Input: part model. Units: mm. Frame: model coordinates. Face numbers are marked on the shaded views. A direction names the side the tool comes from. Round coordinates to 2 decimals unless told otherwise and drop trailing zeros. Write each loop counter-clockwise with the first axis right and the second up, starting at its lowest first coordinate (ties: lowest second). Pieces come first, ordered by that corner, then holes. Notation, with made-up numbers: (57.5, 28) -> (77.5, 28) arc R24 ccw to (77.5, 59) -> close; hole circle Ø4 at (-30.5, -4.75). An arc over 180 degrees is marked (long way). Use CSV: the item, a comma, the result in double quotes.
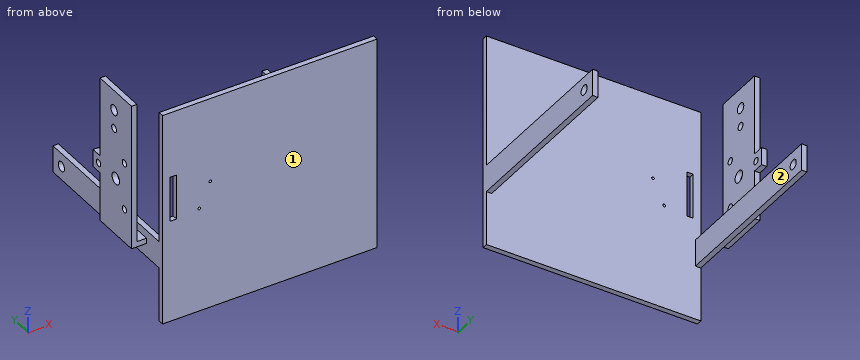
```python
from build123d import *

# Parameters (mm, degrees)
SKETCH1_W                 = 199
SKETCH1_H                 = 199
BOSS_EXTRUDE1_DEPTH       = 5
SKETCH2_W                 = 5
SKETCH2_H                 = 25
BOSS_EXTRUDE2_DEPTH       = 18.8
SKETCH3_W                 = 5
SKETCH3_H                 = 25
BOSS_EXTRUDE3_DEPTH       = 46.4
SKETCH4_W                 = 5
SKETCH4_H                 = 25
BOSS_EXTRUDE4_DEPTH       = 91.8
SKETCH5_W                 = 5
SKETCH5_H                 = 25
BOSS_EXTRUDE5_DEPTH       = 157
SKETCH6_R                 = 4.5
CUT_EXTRUDE1_DEPTH        = 325.724498614
SKETCH8_W                 = 5
SKETCH8_H                 = 46.4
BOSS_EXTRUDE6_DEPTH       = 13.9
SKETCH9_W                 = 5
SKETCH9_H                 = 46.4
BOSS_EXTRUDE7_DEPTH       = 131
SKETCH11_W                = 16.3
SKETCH11_H                = 10.35
BOSS_EXTRUDE8_DEPTH       = 5
SKETCH10_R                = 5.5
SKETCH10_R_2              = 3.15
CUT_EXTRUDE2_DEPTH        = 5
SKETCH12_W                = 6
SKETCH12_H                = 42
CUT_EXTRUDE3_DEPTH        = 5
SKETCH17_R                = 3.5
CUT_EXTRUDE7_DEPTH        = 9
M3X0_5_TAPPED_HOLE1_D     = 2.5
M3X0_5_TAPPED_HOLE1_DEPTH = 7.5
M3X0_5_TAPPED_HOLE1_TIP   = 0.751075774
SKETCH20_R                = 4.7625
CUT_EXTRUDE8_DEPTH        = 10


with BuildPart() as part:
    # Sketch1 → Boss-Extrude1 (new body)
    with BuildSketch(Plane(origin=(0, 0, 0), x_dir=(1, 0, 0), z_dir=(0, 1, 0))):
        with Locations((99.5, -99.5)):
            Rectangle(SKETCH1_W, SKETCH1_H)
    extrude(amount=BOSS_EXTRUDE1_DEPTH)

    # Sketch2 → Boss-Extrude2 (add)
    with BuildSketch(Plane(origin=(0, 5, 0), x_dir=(1, 0, 0), z_dir=(0, 1, 0))):
        with Locations((2.5, -63)):
            Rectangle(SKETCH2_W, SKETCH2_H)
    extrude(amount=BOSS_EXTRUDE2_DEPTH)

    # Sketch3 → Boss-Extrude3 (add)
    with BuildSketch(Plane(origin=(0, 23.8, 0), x_dir=(1, 0, 0), z_dir=(0, 1, 0))):
        with Locations((2.5, -63)):
            Rectangle(SKETCH3_W, SKETCH3_H)
    extrude(amount=BOSS_EXTRUDE3_DEPTH)

    # Sketch4 → Boss-Extrude4 (add)
    with BuildSketch(Plane(origin=(0, 70.2, 0), x_dir=(1, 0, 0), z_dir=(0, 1, 0))):
        with Locations((2.5, -63)):
            Rectangle(SKETCH4_W, SKETCH4_H)
    extrude(amount=BOSS_EXTRUDE4_DEPTH)

    # Sketch5 → Boss-Extrude5 (add)
    with BuildSketch(Plane(origin=(0, 5, 0), x_dir=(1, 0, 0), z_dir=(0, 1, 0))):
        with Locations((196.5, -63)):
            Rectangle(SKETCH5_W, SKETCH5_H)
    extrude(amount=BOSS_EXTRUDE5_DEPTH)

    # Sketch6 → Cut-Extrude1 (cut, through all)
    with BuildSketch(Plane.ZY):
        with Locations((63, 149.5)):
            Circle(SKETCH6_R)
    extrude(amount=-CUT_EXTRUDE1_DEPTH, mode=Mode.SUBTRACT)

    # Sketch8 → Boss-Extrude6 (add)
    with BuildSketch(Plane.ZY):
        with Locations((65.5, 47)):
            Rectangle(SKETCH8_W, SKETCH8_H)
    extrude(amount=BOSS_EXTRUDE6_DEPTH)

    # Sketch9 → Boss-Extrude7 (add)
    with BuildSketch(Plane.XY.offset(68)):
        with Locations((-11.4, 47)):
            Rectangle(SKETCH9_W, SKETCH9_H)
    extrude(amount=BOSS_EXTRUDE7_DEPTH)

    # Sketch11 → Boss-Extrude8 (add)
    with BuildSketch(Plane.ZY.offset(13.9)):
        with Locations((116.5, 75.375)):
            Rectangle(SKETCH11_W, SKETCH11_H)
    extrude(amount=-BOSS_EXTRUDE8_DEPTH)

    # Sketch10 → Cut-Extrude2 (cut)
    with BuildSketch(Plane.ZY.offset(13.9)):
        with Locations((116.5, 47)):
            Circle(SKETCH10_R)
        with Locations((116.5, 72.4)):
            Circle(SKETCH10_R_2)
        with Locations((138.497045256, 34.3)):
            Circle(SKETCH10_R_2)
        with Locations((94.502954744, 34.3)):
            Circle(SKETCH10_R_2)
    extrude(amount=-CUT_EXTRUDE2_DEPTH, mode=Mode.SUBTRACT)

    # Sketch12 → Cut-Extrude3 (cut)
    with BuildSketch(Plane(origin=(0, 5, 0), x_dir=(1, 0, 0), z_dir=(0, 1, 0))):
        with Locations((10, -116.5)):
            Rectangle(SKETCH12_W, SKETCH12_H)
    extrude(amount=-CUT_EXTRUDE3_DEPTH, mode=Mode.SUBTRACT)

    # Sketch17 → Cut-Extrude7 (cut)
    with BuildSketch(Plane.ZY.offset(13.9)):
        with Locations((162.886026442, 49.5625)):
            Circle(SKETCH17_R)
    extrude(amount=-CUT_EXTRUDE7_DEPTH, mode=Mode.SUBTRACT)

    # M3x0.5 Tapped Hole1
    with Locations(Plane(origin=(0, 5, 0), x_dir=(1, 0, 0), z_dir=(0, 1, 0))):
        with Locations((34, -97.8), (44.31875, -120)):
            Hole(M3X0_5_TAPPED_HOLE1_D / 2, depth=M3X0_5_TAPPED_HOLE1_DEPTH)
            with Locations((0, 0, -(M3X0_5_TAPPED_HOLE1_DEPTH + M3X0_5_TAPPED_HOLE1_TIP / 2))):  # 118° drill point
                Cone(0, M3X0_5_TAPPED_HOLE1_D / 2, M3X0_5_TAPPED_HOLE1_TIP, mode=Mode.SUBTRACT)

    # Sketch20 → Cut-Extrude8 (cut)
    with BuildSketch(Plane.ZY.offset(13.9)):
        with Locations((180.348526442, 49.5625)):
            Circle(SKETCH20_R)
    extrude(amount=-CUT_EXTRUDE8_DEPTH, mode=Mode.SUBTRACT)


solid = part.part
```
Item 1: Section query C-C on z = 87. Return the cut outline in (x, y).
Worked answers:
outline,"(-13.9, 23.8) -> (-8.9, 23.8) -> (-8.9, 70.2) -> (-13.9, 70.2) -> close; (0, 0) -> (199, 0) -> (199, 5) -> (0, 5) -> close"
Item 2: First-contact query: pin 1 Ø1.5 at (x, y) = (-11.5, 77.5) entering from -Z; pin 2 Ø5 at (y, z) = (34.3, 94.5) entering from -X; pin 3 Ø1.5 at (x, y) = (3.5, 59) entering from -Z; pin 4 Ø1.5 at (x, z) = (139.5, 127) entering from +Y. Flat tips, straight axial feed; report the tip coordinate or a pass-through.
Worked answers:
pin 1,"stops at z = 108.35"
pin 2,"passes through"
pin 3,"stops at z = 50.5"
pin 4,"stops at y = 5"
Item 3: Section query A-A on y = 34.3. Return the cut outline in (x, z).
Worked answers:
outline,"(-13.9, 63) -> (0, 63) -> (0, 50.5) -> (5, 50.5) -> (5, 75.5) -> (0, 75.5) -> (0, 68) -> (-8.9, 68) -> (-8.9, 91.35) -> (-13.9, 91.35) -> close; (-13.9, 97.65) -> (-8.9, 97.65) -> (-8.9, 135.35) -> (-13.9, 135.35) -> close; (-13.9, 141.65) -> (-8.9, 141.65) -> (-8.9, 199) -> (-13.9, 199) -> close; (194, 50.5) -> (199, 50.5) -> (199, 75.5) -> (194, 75.5) -> close"
Item 4: Section query D-D on x = 180. Return the cut outline in (y, z).
Worked answers:
outline,"(0, 0) -> (5, 0) -> (5, 199) -> (0, 199) -> close"
Item 5: Set-up query: the marked faces 1 and 2. Return all of +Z, -Z, +X, -X, +Y, -Y with unobstructed straight access to the full face (end or side cutting, diameter ignored); none if empty.
Worked answers:
face 1,"+Z, -Z, +X, -X, -Y"
face 2,"+Z, -Z, +Y"
Item 6: Section query B-B on y = 59.5. Return the cut outline in (x, z), plus the area to 4 significant figures.
Worked answers:
outline,"(-13.9, 63) -> (0, 63) -> (0, 50.5) -> (5, 50.5) -> (5, 75.5) -> (0, 75.5) -> (0, 68) -> (-8.9, 68) -> (-8.9, 199) -> (-13.9, 199) -> close; (194, 50.5) -> (199, 50.5) -> (199, 75.5) -> (194, 75.5) -> close"
area,"974.5 mm²"
Item 7: Line query: line 1 (X direction, y = 2.9, z = 97.8); line 2 (X direction, y = 40.5, z = 58); line 3 (Y direction, x = 2.7, z = 63). Output: solid intervals per line, ascending.
Worked answers:
line 1,"x = 0 to 7, 13 to 32.75, 35.25 to 199"
line 2,"x = 0 to 5, 194 to 199"
line 3,"y = 0 to 145, 154 to 162"
